Check sheet for the modelled part. Datum: model origin and axes. Units: mm. A direction names the side the tool comes from. Coordinates: 2 decimals unless noted, no trailing zeros. Order: outer loops, then holes, each group sorted by start corner. A loop starts at its lowest first (then second) coordinate and runs counter-clockwise, first axis right, second up.
from build123d import *

# Parameters (mm, degrees)
F1_DEPTH = 100
F2_W     = 70
F2_H     = 20
F3_DEPTH = 252
F4_W     = 137.891564
F4_H     = 4.743971
F5_DEPTH = 40
F6_R     = 23.773189
F6_R_2   = 21.492651
F6_R_3   = 20.679115
F6_R_4   = 11.883374
F6_R_5   = 6.549136
F6_R_6   = 16.088576
F6_R_7   = 18.070401
F6_R_8   = 10.573912
F6_R_9   = 6.113208
F6_R_10  = 8.058557
F6_R_11  = 2.767323
F6_R_12  = 4.981171
F6_R_13  = 4.462164
F6_R_14  = 5.644248
F6_R_15  = 3.500411
F7_DEPTH = 357


with BuildPart() as f1:
    # F0 (on Front) → F1 (new body)
    with BuildSketch(Plane.XZ):
        with BuildLine():
            Line((179.331843, 175), (-70.668157, 175))
            ThreePointArc((-70.668157, 175), (-154.979102, -20.939428), (-302.511929, -175))
            Line((-302.511929, -175), (133.648471, -175))
            ThreePointArc((133.648471, -175), (130.170691, 3.43532), (179.331843, 175))
        make_face()
    extrude(amount=F1_DEPTH)

    # F2 (on face) → F3 (cut)
    with BuildSketch(Plane.XY.offset(175)):
        with Locations((29.123203, -60)):
            Rectangle(F2_W, F2_H)
    extrude(amount=-F3_DEPTH, mode=Mode.SUBTRACT)

    # F4 (on face) → F5 (join)
    with BuildSketch(Plane.XZ.offset(100)):
        with Locations((42.198492, 87.131027)):
            Rectangle(F4_W, F4_H)
    extrude(amount=-F5_DEPTH)

    # F6 (on face) → F7 (cut)
    with BuildSketch(Plane.XZ.offset(100)):
        with Locations((-70.998937, 29.887047)):
            Circle(F6_R)
        with Locations((-36.130711, -14.39006)):
            Circle(F6_R_2)
        with Locations((-72.105862, -57.560239)):
            Circle(F6_R_3)
        with Locations((-96.458264, -11.069277)):
            Circle(F6_R_4)
        with Locations((0, -32.654367)):
            Circle(F6_R_5)
        with Locations((-19.526798, -58.667168)):
            Circle(F6_R_6)
        with Locations((10.913723, 0)):
            Circle(F6_R_7)
        with Locations((-27.828749, 33.20783)):
            Circle(F6_R_8)
        with Locations((-9.564446, 26.012801)):
            Circle(F6_R_9)
        with Locations((-68.785071, -5.534639)):
            Circle(F6_R_10)
        with Locations((-73.212788, -28.780119)):
            Circle(F6_R_11)
        with Locations((-38.344566, -45.937501)):
            Circle(F6_R_12)
        with Locations((-41.665345, -68.629518)):
            Circle(F6_R_13)
        with Locations((-17.866395, 13.283132)):
            Circle(F6_R_14)
        with Locations((-36.130711, 15.496987)):
            Circle(F6_R_15)
    extrude(amount=-F7_DEPTH, mode=Mode.SUBTRACT)


solid = f1.part
(1) Cross-section at A-A (z = 108). Enter the section's corners in (x, y).
Filled in:
outline: (-90.36, -100) - (153.46, -100) - (153.46, 0) - (-90.36, 0) - close; hole (-5.88, -70) - (64.12, -70) - (64.12, -50) - (-5.88, -50) - close
(2) Tool access check on faces 1 (the cylindrical face through (-85.124, -50.7, -7.5)), 2 (the flat face through (29, -70, 133)), 3 (the flat face through (64.123, -60, 51)). Record the directions out of +Z, -Z, +X, -X, +Y, -Y that give a thin tool (end or side, any length) a straight path to the whole face; none if there is none.
Filled in:
face 1: +Y, -Y
face 2: +Z
face 3: none
(3) Release check for a two-part mould opening along Z. For faces 4 (the cylindrical face through (-15.67, -50.7, 26.28)), 5 (the flat face through (-87, -49, -175)), 6 (the flat face through (56, -49, 175)) record: +Z half, -Z half, draft (parallel to the pull), parting line (faces both ways), or undercut.
Filled in:
face 4: undercut
face 5: -Z half
face 6: +Z half
(4) Thickness scan on probe 1 along Z at (x, y) = (-21.5, -43); probe 2 along Z at (x, y) = (0, -28.5); probe 3 along X at (y, z) = (-61.5, 17). Record the ranges inside material, lowest first.
Filled in:
probe 1: z = -175 to -74.63, -42.7 to -30.13, 1.35 to 8.96, 17.6 to 24.74, 41.68 to 175
probe 2: z = -175 to -39.2, -26.11 to -14.4, 14.4 to 175
probe 3: x = -131.82 to -90.98, -51.02 to -39.29, -32.97 to -22.11, -13.62 to -5.88, 64.12 to 132.1
(5) Cross-section at B-B (y = -55). Count the separate pieces of the cut face and the enclosed holes in it, and give its area (3 significant figures).
Filled in:
separate pieces: 1
enclosed holes: 11
area: 78,700 mm2
(6) Cross-section at D-D (x = -244). Enter the section's corners in (y, z), and give its area (3 significant figures).
Filled in:
outline: (-100, -175) - (0, -175) - (0, -126.54) - (-100, -126.54) - close
area: 4,850 mm2
(7) Go/stop test with a flat-tipped pin: P1, Ø3, axis at y = -60, z = -123.5, coming from the -X side. Record where the tip stops, or that it passes through.
Filled in:
P1: stops at x = -242.37
